from build123d import *

# Parameters (mm, degrees)
SKETCH_R             = 17.86
PAD_DEPTH            = 1.6
SKETCH001_R          = 4.765
PAD001_DEPTH         = 7.96
SKETCH002_R          = 2.15
POCKET_DEPTH         = 9.561
SKETCH003_R          = 1.6
POCKET001_DEPTH      = 5
POCKET001_DEPTH_BACK = -5
SKETCH004_R          = 2.15
POCKET002_DEPTH      = 112.385713
POLARPATTERN_COUNT   = 6


with BuildPart() as part:
    # Sketch → Pad (new body)
    with BuildSketch(Plane.XY):
        Circle(SKETCH_R)
    extrude(amount=PAD_DEPTH)

    # Sketch001 (on Face3 of Pad) → Pad001 (join)
    with BuildSketch(Plane.XY.offset(1.6)):
        Circle(SKETCH001_R)
    extrude(amount=PAD001_DEPTH)

    # Sketch002 (on Face5 of Pad001) → Pocket (cut, through all)
    with BuildSketch(Plane.XY.offset(9.56)):
        Circle(SKETCH002_R)
    extrude(amount=-POCKET_DEPTH, mode=Mode.SUBTRACT)

    # Sketch003 (on DatumPlane) → Pocket001 (cut, two sides)
    with BuildSketch(Plane(origin=(0, 0, 0), x_dir=(0.866025, 0.5, 0), z_dir=(0.5, -0.866025, 0))) as pocket001_sk:
        with Locations((0, 5.57)):
            Circle(SKETCH003_R)
    extrude(amount=-POCKET001_DEPTH, mode=Mode.SUBTRACT)
    extrude(pocket001_sk.sketch, amount=-POCKET001_DEPTH_BACK, mode=Mode.SUBTRACT)

    # Sketch004 → Pocket002 (cut, through all)
    with BuildSketch(Plane.XY):
        with Locations((0, 12.7)):
            Circle(SKETCH004_R)
    pocket002 = extrude(amount=POCKET002_DEPTH, mode=Mode.SUBTRACT)

    # PolarPattern: Pocket002 ×6 about axis
    polarpattern_axis = Axis((0, 0, 0), (0, 0, 1))
    for i in range(1, POLARPATTERN_COUNT):
        add(pocket002.rotate(polarpattern_axis, i * 360 / POLARPATTERN_COUNT), mode=Mode.SUBTRACT)


solid = part.part
Design review of the part built by this model. Coordinates are the model's own, in mm. A direction names the side the tool comes from. Give positions to 0.01 mm unless a question says otherwise; leave off trailing zeros. Order: outer loops, then holes, each group sorted by start corner. A loop starts at its lowest first (then second) coordinate and runs counter-clockwise, first axis right, second up.
1. Tool access review of faces 4 (the flat face through (4, -4, 1.6)), 5 (the cylindrical face through (-2.923, 1.867, 5.64)): name each direction out of +Z, -Z, +X, -X, +Y, -Y from which nothing blocks a thin tool from reaching the whole face with its end or side.
Solution:
face 4: +Z
face 5: none
2. Add section B-B, the plane y = 6.35. State the section outline as (x, z) points, then the cut area to 3 significant figures.
Solution:
outline: (-16.69, 0) - (-13.15, 0) - (-13.15, 1.6) - (-16.69, 1.6) - close; (-8.85, 0) - (8.85, 0) - (8.85, 1.6) - (-8.85, 1.6) - close; (13.15, 0) - (16.69, 0) - (16.69, 1.6) - (13.15, 1.6) - close
area: 39.7 mm2
3. To check wall thickness, follow L1, parallel to Y at x = 0, z = 0.4; L2, parallel to Y at x = 0, z = 8 (3 decimals); L3, parallel to Z at x = -2.5, y = -11.5. State the ranges of each line that lie inside material, in increasing order.
Solution:
L1: y = -17.86 to -14.85, -10.55 to -2.15, 2.15 to 10.55, 14.85 to 17.86
L2: y = -4.765 to -2.15, 2.15 to 4.765
L3: z = 0 to 1.6
4. Mouldability with a two-part tool opening along Y and no side actions: class faces 1 (the flat face through (2.1, -1, 9.56)), 2 (the cylindrical face through (-3.872, -17.435, 0.789)), 3 (the cylindrical face through (0.155, -3.465, 5.64)) as +Y half, -Y half, draft (parallel to the pull), parting line (faces both ways), or undercut.
Solution:
face 1: draft
face 2: parting line
face 3: undercut
5. Add section C-C, the plane z = 2.5. State the section outline as (x, y) points (3 decimals).
Solution:
outline: circle Ø9.53 at (0, 0); hole circle Ø4.3 at (0, 0)
6. Add section D-D, the plane x = -10.5. State the section outline as (y, z) points.
Solution:
outline: (-14.45, 0) - (-8.44, 0) - (-8.44, 1.6) - (-14.45, 1.6) - close; (-4.26, 0) - (4.26, 0) - (4.26, 1.6) - (-4.26, 1.6) - close; (8.44, 0) - (14.45, 0) - (14.45, 1.6) - (8.44, 1.6) - close
7. Add section A-A, the plane y = 0. State the section outline as (x, z) points (3 decimals), then the cut area to 3 significant figures.
Solution:
outline: (-17.86, 0) - (-2.15, 0) - (-2.15, 9.56) - (-4.765, 9.56) - (-4.765, 1.6) - (-17.86, 1.6) - close; (2.15, 0) - (17.86, 0) - (17.86, 1.6) - (4.765, 1.6) - (4.765, 9.56) - (2.15, 9.56) - close
area: 91.9 mm2
8. For pin 1 Ø4 at (y, z) = (-6, 5.5) entering from -X; pin 2 Ø5 at (x, z) = (5.5, 5) entering from +Y; pin 3 Ø3.5 at (x, y) = (0, 0) entering from -Z; pin 4 Ø5 at (x, y) = (0, -12.7) entering from +Z, all flat-tipped, find the tip position at first contact; note any pin that passes through.
Solution:
pin 1: stops at x = -2.59
pin 2: stops at y = 3.7
pin 3: passes through
pin 4: stops at z = 1.6
